Could you check a few things on this model? Use its own coordinates, in mm. A direction names the side the tool comes from. Give positions to 0.01 mm unless a question says otherwise; leave off trailing zeros. Write each loop counter-clockwise with the first axis right and the second up, starting at its lowest first coordinate (ties: lowest second). Pieces come first, ordered by that corner, then holes. Notation, with made-up numbers: (45, -31.75) - (84, -31.75) arc R27 ccw to (84, -4.75) - close; hole circle Ø9 at (-19.5, 42). An arc over 180 degrees is marked (long way). Answer in a Markdown table with one row per item.
from build123d import *

# Parameters (mm, degrees)
F0_R     = 1.5
F1_DEPTH = 10
F3_DEPTH = 8
F5_DEPTH = 5
F6_R     = 1.5
F7_DEPTH = 4.001
F6_R_2   = 2.5
F8_DEPTH = 1


with BuildPart() as f1:
    # F0 (on Top) → F1 (new body)
    with BuildSketch(Plane.XY):
        with BuildLine():
            Line((10, -5), (10, 5))
            Line((10, 5), (3, 5))
            Line((3, 5), (3, 7))
            Line((3, 7), (-3, 7))
            Line((-3, 7), (-3, 5))
            Line((-3, 5), (-10, 5))
            Line((-10, 5), (-10, -5))
            Line((-10, -5), (0, -5))
            Line((0, -5), (0, -4))
            ThreePointArc((0, -4), (-3, -1), (0, 2))
            Line((0, 2), (0, 3))
            Line((0, 3), (4, 3))
            Line((4, 3), (4, -5))
            Line((4, -5), (10, -5))
        make_face()
        with Locations((-7, -1)):
            Circle(F0_R, mode=Mode.SUBTRACT)
        with Locations((7, -1)):
            Circle(F0_R, mode=Mode.SUBTRACT)
        with BuildLine():
            Line((0, -5), (4, -5))
            Line((4, -5), (4, 3))
            Line((4, 3), (0, 3))
            Line((0, 3), (0, 2))
            ThreePointArc((0, 2), (2.1213203436, 1.1213203436), (3, -1))
            ThreePointArc((3, -1), (2.1213203436, -3.1213203436), (0, -4))
            Line((0, -4), (0, -5))
        make_face()
        with BuildLine():
            Line((0, -2.5), (0, -4))
            ThreePointArc((0, -4), (2.1213203436, -3.1213203436), (3, -1))
            ThreePointArc((3, -1), (2.1213203436, 1.1213203436), (0, 2))
            Line((0, 2), (0, 0.5))
            ThreePointArc((0, 0.5), (1.0606601718, 0.0606601718), (1.5, -1))
            ThreePointArc((1.5, -1), (1.0606601718, -2.0606601718), (0, -2.5))
        make_face()
        with BuildLine():
            ThreePointArc((0, 2), (-3, -1), (0, -4))
            Line((0, -4), (0, -2.5))
            ThreePointArc((0, -2.5), (-1.5, -1), (0, 0.5))
            Line((0, 0.5), (0, 2))
        make_face()
    extrude(amount=-F1_DEPTH)

    # F0 (on Top) → F2 (revolve, cut)
    with BuildSketch(Plane.XY):
        with BuildLine():
            Line((0, -5), (4, -5))
            Line((4, -5), (4, 3))
            Line((4, 3), (0, 3))
            Line((0, 3), (0, 2))
            ThreePointArc((0, 2), (2.1213203436, 1.1213203436), (3, -1))
            ThreePointArc((3, -1), (2.1213203436, -3.1213203436), (0, -4))
            Line((0, -4), (0, -5))
        make_face()
        with BuildLine():
            Line((0, -2.5), (0, -4))
            ThreePointArc((0, -4), (2.1213203436, -3.1213203436), (3, -1))
            ThreePointArc((3, -1), (2.1213203436, 1.1213203436), (0, 2))
            Line((0, 2), (0, 0.5))
            ThreePointArc((0, 0.5), (1.0606601718, 0.0606601718), (1.5, -1))
            ThreePointArc((1.5, -1), (1.0606601718, -2.0606601718), (0, -2.5))
        make_face()
    revolve(axis=Axis((0, -1, 0), (0, 1, 0)), mode=Mode.SUBTRACT)

    # F0 (on Top) → F3 (cut)
    with BuildSketch(Plane.XY):
        with BuildLine():
            ThreePointArc((0, 2), (-3, -1), (0, -4))
            Line((0, -4), (0, -2.5))
            ThreePointArc((0, -2.5), (-1.5, -1), (0, 0.5))
            Line((0, 0.5), (0, 2))
        make_face()
        with BuildLine():
            Line((0, -2.5), (0, -4))
            ThreePointArc((0, -4), (2.1213203436, -3.1213203436), (3, -1))
            ThreePointArc((3, -1), (2.1213203436, 1.1213203436), (0, 2))
            Line((0, 2), (0, 0.5))
            ThreePointArc((0, 0.5), (1.0606601718, 0.0606601718), (1.5, -1))
            ThreePointArc((1.5, -1), (1.0606601718, -2.0606601718), (0, -2.5))
        make_face()
    extrude(amount=-F3_DEPTH, mode=Mode.SUBTRACT)

    # F4 (on face) → F5 (join)
    with BuildSketch(Plane.XY):
        Polygon((-10, 5), (-10, 3), (0, 3), (4, 3), (10, 3), (10, 5), (3, 5), (3, 7), (-3, 7), (-3, 5), align=None)
    extrude(amount=F5_DEPTH)

    # F6 (on face) → F7 (cut, through all)
    with BuildSketch(Plane.XZ.offset(-3)):
        Circle(F6_R)
    extrude(amount=-F7_DEPTH, mode=Mode.SUBTRACT)

    # F6 (on face) → F8 (cut)
    with BuildSketch(Plane.XZ.offset(-3)):
        Circle(F6_R_2)
        Circle(F6_R, mode=Mode.SUBTRACT)
    extrude(amount=-F8_DEPTH, mode=Mode.SUBTRACT)


solid = f1.part
1) Imagine slicing it at B-B (x = -7). List the corners of the cut face in (y, z) for me, then the cut area to 3 significant figures.
Check values:
| item | result |
|---|---|
| outline | (-5, -10) - (-2.5, -10) - (-2.5, 0) - (-5, 0) - close; (0.5, -10) - (5, -10) - (5, 5) - (3, 5) - (3, 0) - (0.5, 0) - close |
| area | 80.0 mm2 |
2) Will these pins go through, and if not, where does the flat tip stop? P1, Ø5, axis at x = -6, y = 1, coming from the +Z side; P2, Ø2, axis at x = 7.5, z = -5.5, coming from the +Y side; P3, Ø3.5, axis at x = 7, y = -1, coming from the +Z side; P4, Ø1, axis at y = 6.5, z = -6, coming from the -X side.
Check values:
| item | result |
|---|---|
| P1 | stops at z = 5 |
| P2 | stops at y = 5 |
| P3 | stops at z = 0 |
| P4 | stops at x = -3 |
3) We'd pull the mould along Z, two halves only. Please class faces 1 (the face through (0, 1, -10)), 2 (the face through (0, 4, -2)), 3 (the face through (3, 6, -3)), 4 (the face through (-0.54, 3.49, -2.44)): +Z half, -Z half, draft (parallel to the pull), parting line (faces both ways), or undercut.
Check values:
| item | result |
|---|---|
| face 1 | -Z half |
| face 2 | undercut |
| face 3 | draft |
| face 4 | undercut |
4) Imagine slicing it at D-D (y = 2.5). List the corners of the cut face in (x, z) for me.
Check values:
| item | result |
|---|---|
| outline | (-10, -10) - (10, -10) - (10, 0) - (4, 0) arc R4 cw to (-4, 0) - (-10, 0) - close |
5) On a 3-axis mill with a long thin cutter (end or side, diameter ignored), from which of +Z, -Z, +X, -X, +Y, -Y can I reach the whole of each face in a straight line? I mean faces 5 (the face through (-3, 6, -3)), 6 (the face through (0, 3, 3)), 7 (the face through (7, 5, -3)). Say none if no direction works.
Check values:
| item | result |
|---|---|
| face 5 | +Z, -Z, -X, +Y |
| face 6 | +Z, -Y |
| face 7 | +Z, -Z, +X, +Y |
6) If I drill on line 1 (Y direction, x = 7, z = -5); line 2 (Z direction, x = 0, y = 5.35); line 3 (Z direction, x = -5, y = 1), over which ranges is the centre line in solid material (lowest first)?
Check values:
| item | result |
|---|---|
| line 1 | y = -5 to -2.5, 0.5 to 5 |
| line 2 | z = -10 to -1.5, 1.5 to 5 |
| line 3 | z = -10 to 0 |
7) Imagine slicing it at C-C (x = 0.25). List the corners of the cut face in (y, z) for me, then the cut area to 3 significant figures.
Check values:
| item | result |
|---|---|
| outline | (-5, -10) - (-2.48, -10) - (-2.48, -8) - (-3.99, -8) - (-3.99, -3.99) - (-5, -3.99) - close; (0.48, -10) - (7, -10) - (7, -1.48) - (4, -1.48) - (4, -2.49) - (3, -2.49) - (3, -3.99) - (1.99, -3.99) - (1.99, -8) - (0.48, -8) - close; (3, 2.49) - (4, 2.49) - (4, 1.48) - (7, 1.48) - (7, 5) - (3, 5) - close |
| area | 64.3 mm2 |
8) Imagine slicing it at A-A (z = -7.5). List the corners of the cut face in (x, y) for me, then the cut area to 3 significant figures.
Check values:
| item | result |
|---|---|
| outline | (-10, -5) - (10, -5) - (10, 5) - (3, 5) - (3, 7) - (-3, 7) - (-3, 5) - (-10, 5) - close; hole circle Ø3 at (-7, -1); hole circle Ø6 at (0, -1); hole circle Ø3 at (7, -1) |
| area | 170 mm2 |
